Read the model definition and answer for the solid it produces. Units are mm, in the model's axes. Coordinates: 2 decimals unless noted, no trailing zeros. Order: outer loops, then holes, each group sorted by start corner. A loop starts at its lowest first (then second) coordinate and runs counter-clockwise, first axis right, second up. Notation, with made-up numbers: (-3.5, -13) -> (37.5, -13) arc R25 ccw to (37.5, 15) -> close; hole circle Ø8 at (87, -40). An arc over 180 degrees is marked (long way). Answer as a JSON object with one key per item and string values. Group by question number.
1) Section C-C on x = 2.25 is taken. Determine the outline of the cut face in (y, z).
2) Given pin 1 (4 mm diameter, centred on x = 0.5, z = -17, fed in from +Y); pin 2 (4 mm diameter, centred on x = -4, y = 460.5, fed in from +Z); pin 3 (2 mm diameter, centred on x = -1.5, z = -55, fed in from +Y), each flat-ended and moving along its own axis, determine where each tip first touches the part or whether it passes through.
3) Consider L1, parallel to Z at x = -4, y = 88.5; L2, parallel to Z at x = 0, y = 499.5. Determine where each line is inside the solid, lowest interval first.
Autodesk Inventor part; units mm, degrees
sketch "草圖1" plane through (0, 0, 0) normal (1, 0, 0) x (0, 1, 0)
  line L0 (0, 0) -> (674.096, -106.071)
  line L1 (0, 0) -> (614.096, 0)
  line L2 (674.096, -106.071) -> (674.096, -60)
  line L3 (674.096, -106.071) -> (0, -106.071) construction
  line L4 (0, 0) -> (0, -106.071)
  arc A0 (674.096, -60) -> (614.096, 0) centre (614.096, -60) ccw
  dimension "d0" = 106.071
  dimension "d1" = 674.096
  dimension "d2" = 60
extrude "擠出1" add sketch "草圖1" along normal mid plane 10
ref_plane "工作平面1" through (0, 674.096, 0) normal (0, 1, 0) x (-1, 0, 0)
fillet "圓角1" radius 5 6 edges at (-5, 656.5224, -17.5736) (-5, 307.048, 0) (-5, 674.096, -83.0355) (5, 307.048, 0) (5, 674.096, -83.0355) (5, 656.5224, -17.5736)
properties part number "路徑"
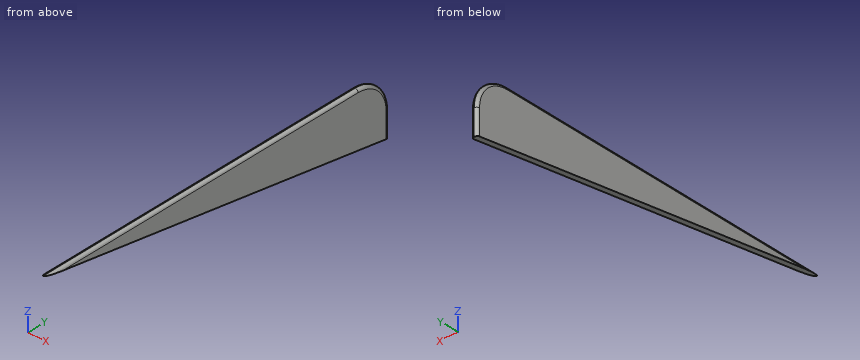
Worked answers:
{
 "1": {"outline": "(3.4, -0.53) -> (673.56, -105.99) -> (673.56, -60) arc R59.47 ccw to (614.1, -0.53) -> close"},
 "2": {"pin 1": "stops at y = 657.88", "pin 2": "stops at z = -0.42", "pin 3": "stops at y = 673.89"},
 "3": {"L1": "z = -13.93 to -2", "L2": "z = -78.6 to 0"}
}
